Design review of the part built by this model. Coordinates are the model's own, in mm. A direction names the side the tool comes from. Round coordinates to 2 decimals unless told otherwise and drop trailing zeros. Order: outer loops, then holes, each group sorted by start corner. A loop starts at its lowest first (then second) coordinate and runs counter-clockwise, first axis right, second up. Notation, with made-up numbers: M 10,17 L 45,17 A23 cw 45,31 Z; hole C -30.5,71.25 d4. An arc over 180 degrees is marked long. Use a Markdown table: item, result. Add a question column.
(1) To check wall thickness, follow probe 1 along X at (y, z) = (1.6, 3.5); probe 2 along X at (y, z) = (2.3, -2); probe 3 along Z at (x, y) = (26.5, 2.3). State the ranges of each line that lie inside material, in increasing order. Write a range as from..to.
(2) Take a section at A-A (z = 0.25). Write out the cut boundary in (x, y).
(3) The part is to be moulded in two halves that separate along Z. For faces 4 (the face through (-40.8, 1, -3)), 5 (the face through (-35.6, 1, 0)), 6 (the face through (0, 1, 2.3)), 7 (the face through (35.6, 1, 0)), say which applies: released by +Z, released by -Z, zero draft, split by the parting line, or undercut.
(4) For pin 1 (1.5 mm diameter, centred on x = 5, y = 2, fed in from +Z); pin 2 (0.8 mm diameter, centred on y = 1, z = -0.5, fed in from -X); pin 3 (1.3 mm diameter, centred on y = 1, z = 0, fed in from +X), all flat-tipped, find the tip position at first contact; note any pin that passes through.
(5) Take a section at B-B (x = -14). Write out the cut boundary in (y, z), then the cut area to 3 significant figures.
(6) Machinability: for faces 1 (the face through (0, 1, -2.3)), 2 (the face through (39, 1, -1.05)), 3 (the face through (-39, 1, 1.05)), which of the approach directions +Z, -Z, +X, -X, +Y, -Y give a long, thin tool a straight path to every point of the face, cutting with its end or side? Answer none if there is none.
```python
from build123d import *

# Parameters (mm, degrees)
SKETCH1_W         = 67.8
SKETCH1_H         = 4.6
BASE_SHAPE_DEPTH  = 3
MILLING_FILLETS_R = 1


with BuildPart() as part:
    # Sketch1 → Base shape (new body)
    with BuildSketch(Plane(origin=(0, 0, 0), x_dir=(1, 0, 0), z_dir=(0, 1, 0))):
        Rectangle(SKETCH1_W, SKETCH1_H)
        Polygon((-33.9, 4), (-40.8, 4), (-40.8, 1.05), (-37.8, 1.05), (-37.8, 2.3), (-35.6, 2.3), (-35.6, -2.3), (-37.8, -2.3), (-37.8, -1.05), (-40.8, -1.05), (-40.8, -4), (-33.9, -4), (-33.9, -2.3), (-33.9, 2.3), align=None)
        Polygon((40.8, 4), (33.9, 4), (33.9, 2.3), (33.9, -2.3), (33.9, -4), (40.8, -4), (40.8, -1.05), (37.8, -1.05), (37.8, -2.3), (35.6, -2.3), (35.6, 2.3), (37.8, 2.3), (37.8, 1.05), (40.8, 1.05), align=None)
    extrude(amount=BASE_SHAPE_DEPTH)

    # Milling fillets
    milling_fillets_edges = [part.edges().sort_by_distance(p)[0] for p in [
        (-33.9, 1.5, 2.3),
        (-37.8, 1.5, 2.3),
        (-35.6, 1.5, 2.3),
        (-35.6, 1.5, -2.3),
        (-37.8, 1.5, -2.3),
        (-33.9, 1.5, -2.3),
        (33.9, 1.5, -2.3),
        (37.8, 1.5, -2.3),
        (35.6, 1.5, -2.3),
        (35.6, 1.5, 2.3),
        (37.8, 1.5, 2.3),
        (33.9, 1.5, 2.3),
    ]]
    fillet(milling_fillets_edges, radius=MILLING_FILLETS_R)


solid = part.part
```
Verdict:
| question | item | result |
|---|---|---|
| 1 | probe 1 | x = -40.8..-33.9, 33.9..40.8 |
| 1 | probe 2 | x = -40.8..-37.51, -35.89..35.89, 37.51..40.8 |
| 1 | probe 3 | z = -2.3..2.3 |
| 2 | outline | M -35.6,0 L 35.6,0 L 35.6,3 L -35.6,3 Z |
| 3 | face 4 | zero draft |
| 3 | face 5 | undercut |
| 3 | face 6 | released by +Z |
| 3 | face 7 | undercut |
| 4 | pin 1 | stops at z = 2.3 |
| 4 | pin 2 | stops at x = -35.6 |
| 4 | pin 3 | stops at x = 35.6 |
| 5 | outline | M 0,-2.3 L 3,-2.3 L 3,2.3 L 0,2.3 Z |
| 5 | area | 13.8 mm^2 |
| 6 | face 1 | -Z, +Y, -Y |
| 6 | face 2 | +X, +Y, -Y |
| 6 | face 3 | -X, +Y, -Y |
